Work out the finished part from the listing and answer in its coordinate system (mm). Face numbers are marked on the shaded views. A direction names the side the tool comes from. Coordinates: 2 decimals unless noted, no trailing zeros. Write each loop counter-clockwise with the first axis right and the second up, starting at its lowest first coordinate (ties: lowest second). Pieces come first, ordered by that corner, then holes. Notation, with made-up numbers: (-33, 47) - (10, 47) arc R26 ccw to (10, 66) - close; hole circle Ø8 at (-23, -29.5). An arc over 180 degrees is marked (long way). One line per item, written item: value.
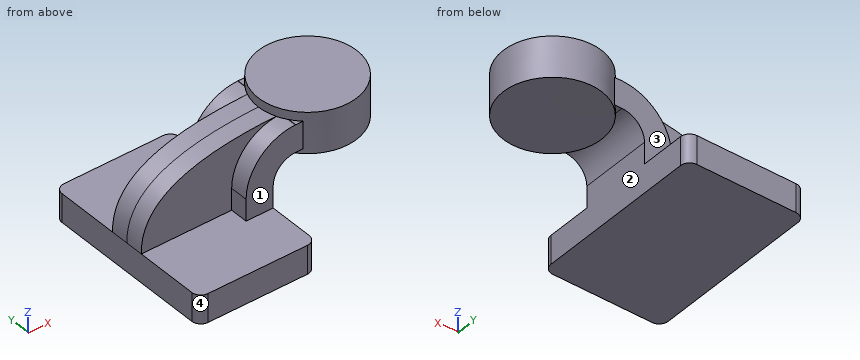
```python
from build123d import *

# Parameters (mm, degrees)
F1_DEPTH = 63.5
F2_DEPTH = 25.4
F4_R     = 6.35
F5_DEPTH = 12.7


with BuildPart() as f1:
    # F0 (on Front) → F1 (new body, symmetric)
    with BuildSketch(Plane.XZ):
        Polygon((-41.275, -10.008192715), (41.275, -10.008192715), (41.275, 10.008192715), (22.225, 10.008192715), (-41.275, 10.008192715), align=None)
    extrude(amount=F1_DEPTH, both=True)

    # F0 (on Front) → F2 (join, symmetric)
    with BuildSketch(Plane.XZ):
        with BuildLine():
            Line((22.225, 10.008192715), (41.275, 10.008192715))
            Line((41.275, 10.008192715), (41.275, 25.136330729))
            ThreePointArc((41.275, 25.136330729), (45.9246798487, 36.3616508803), (57.15, 41.011330729))
            Line((57.15, 41.011330729), (69.4978268266, 41.011330729))
            Line((69.4978268266, 41.011330729), (69.4978268266, 60.061330729))
            Line((69.4978268266, 60.061330729), (57.15, 60.061330729))
            add(Edge.make_bspline(
                [(56.7953338747, 60.0595298514), (56.913590658, 60.0601784283), (57.0318130144, 60.0607785778), (57.15, 60.061330729)],
                knots=[110.1425661044, 110.1425661044, 110.1425661044, 110.1425661044, 110.421000041, 110.421000041, 110.421000041, 110.421000041], degree=3))
            ThreePointArc((56.7953338747, 60.0595298514), (32.3292189947, 49.7063216791), (22.225, 25.136330729))
            Line((22.225, 25.136330729), (22.225, 10.008192715))
        make_face()
        Polygon((69.4978268266, 60.061330729), (69.4978268266, 41.011330729), (85.7105576537, 41.011330729), (85.7214838447, 60.061330729), align=None)
    extrude(amount=F2_DEPTH, both=True)

    # F0 (on Front) → F3 (revolve)
    with BuildSketch(Plane.XZ):
        Polygon((85.7214838447, 60.061330729), (85.7105576537, 41.011330729), (85.7086107135, 37.616807285), (120.2978268266, 37.616807285), (120.2978268266, 66.191807285), (85.725, 66.191807285), align=None)
    revolve(axis=Axis((85.7168053567, 0, 51.904307285), (0.0005735532, 0, 0.9999998355)))

    # F4
    f4_edges = [f1.edges().sort_by_distance(p)[0] for p in [
        (-41.275, -63.5, 0),
        (41.275, -63.5, 0),
        (41.275, 63.5, 0),
        (-41.275, 63.5, 0),
    ]]
    fillet(f4_edges, radius=F4_R)

    # F0 (on Front) → F5 (join, symmetric)
    with BuildSketch(Plane.XZ):
        with BuildLine():
            add(Edge.make_bspline(
                [(-41.275, 10.008192715), (-42.1516341182, 51.9683743999), (10.0154559074, 59.8029665762), (56.7953338747, 60.0595298514)],
                knots=[0, 0, 0, 0, 110.1425661044, 110.1425661044, 110.1425661044, 110.1425661044], degree=3))
            Line((-41.275, 10.008192715), (22.225, 10.008192715))
            Line((22.225, 10.008192715), (22.225, 25.136330729))
            ThreePointArc((22.225, 25.136330729), (32.3292189947, 49.7063216791), (56.7953338747, 60.0595298514))
        make_face()
    extrude(amount=F5_DEPTH, both=True)


solid = f1.part
```
Item 1: Section A-A, the plane z = 7 is taken. Determine the outline of the cut face in (x, y) (3 decimals), then the cut area to 3 significant figures.
Evaluation:
outline: (-41.275, -57.15) arc R6.35 ccw to (-34.925, -63.5) - (34.925, -63.5) arc R6.35 ccw to (41.275, -57.15) - (41.275, 57.15) arc R6.35 ccw to (34.925, 63.5) - (-34.925, 63.5) arc R6.35 ccw to (-41.275, 57.15) - close
area: 10,400 mm2
Item 2: Given pin 1 (10 mm diameter, centred on y = 20, z = 17, fed in from -X) (3 decimals); pin 2 (25 mm diameter, centred on x = 3.5, z = 35, fed in from -Y); pin 3 (4 mm diameter, centred on x = 59, y = 24, fed in from -Z), each flat-ended and moving along its own axis, determine where each tip first touches the part or whether it passes through.
Evaluation:
pin 1: stops at x = 22.225
pin 2: stops at y = -12.7
pin 3: stops at z = 37.65
Item 3: Which of the six approach directions +Z, -Z, +X, -X, +Y, -Y give full straight-line access (tool end or side, diameter ignored) to the marked faces 1, 2, 3 and 4?
Evaluation:
face 1: +Z, -X, -Y
face 2: -Z, +X, +Y, -Y
face 3: +Z, -X, +Y
face 4: +Z, -Z, -X, -Y
Item 4: Section B-B, the plane y = 46 is taken. Determine the outline of the cut face in (x, z) (3 decimals), then the cut area to 3 significant figures.
Evaluation:
outline: (-41.275, -10.008) - (41.275, -10.008) - (41.275, 10.008) - (-41.275, 10.008) - close
area: 1,650 mm2
Item 5: Consider probe 1 along Z at (x, y) = (0.5, 13.5); probe 2 along Z at (x, y) = (62, 18); probe 3 along Y at (x, z) = (61, 48). Determine where each line is inside the solid, lowest interval first.
Evaluation:
probe 1: z = -10.01 to 10.01
probe 2: z = 37.65 to 66.22
probe 3: y = -25.4 to 25.4
